Geometry check sheet. Reference: drawing and pictorial views, mm from the part's lowest x, y, z. A direction names the side the tool comes from. Round coordinates to 2 decimals unless told otherwise and drop trailing zeros. Order: outer loops, then holes, each group sorted by start corner. A loop starts at its lowest first (then second) coordinate and runs counter-clockwise, first axis right, second up. Notation, with made-up numbers: (55, 12.25) -> (104, 12.25) arc R33 ccw to (104, 46.25) -> close; hole circle Ø6 at (-40, 82.5). An arc over 180 degrees is marked (long way). Put each result on its own line as item: value.
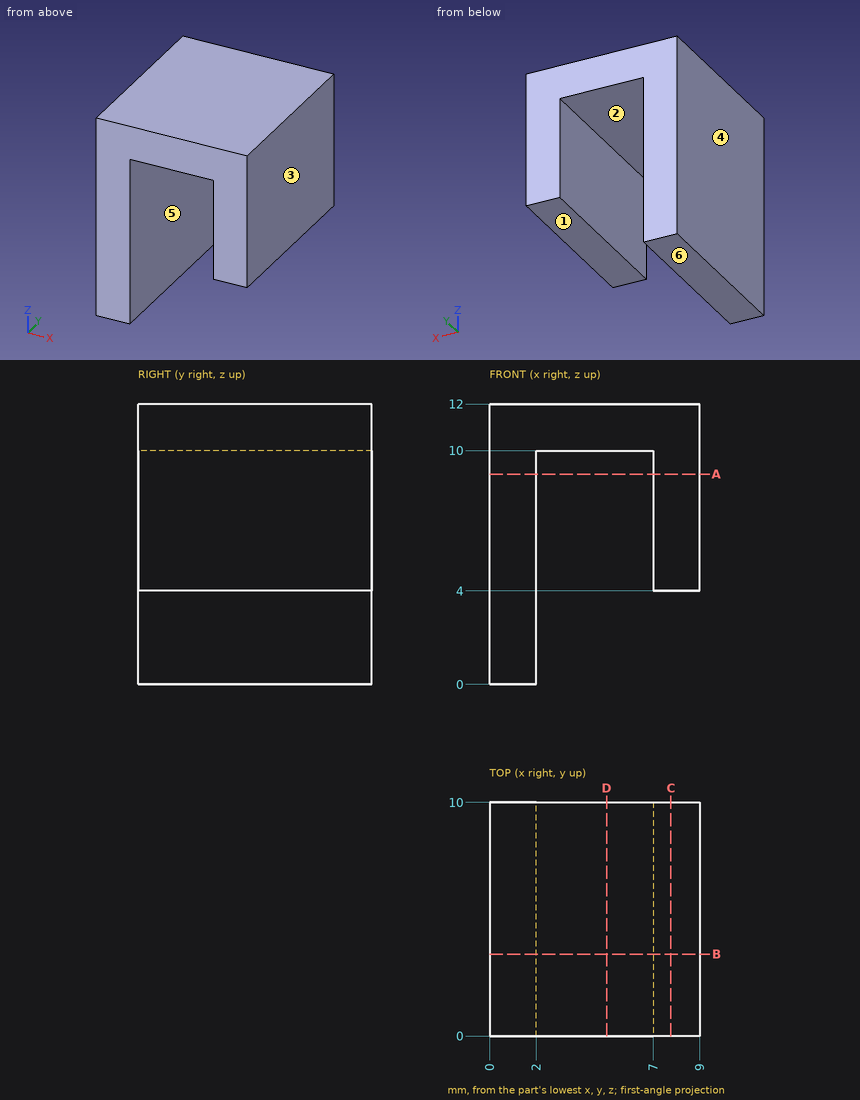
Item 1: Tool access check on the marked faces 5 and 6. Record the directions out of +Z, -Z, +X, -X, +Y, -Y that give a thin tool (end or side, any length) a straight path to the whole face; none if there is none.
Geometry check:
face 5: -Z, +Y, -Y
face 6: -Z, +X, -X, +Y, -Y
Item 2: Release check for a two-part mould opening along X. For the marked faces 1, 2, 3 and 4 record: pulls with the +X half, pulls with the -X half, needs draft (parallel to the pull), parting line crosses it, or undercut.
Geometry check:
face 1: needs draft
face 2: undercut
face 3: pulls with the +X half
face 4: pulls with the -X half
Item 3: Sectioned sample at D-D, the plane x = 5. Record the boundary of the cut face in (y, z).
Geometry check:
outline: (0, 10) -> (10, 10) -> (10, 12) -> (0, 12) -> close
Item 4: Material ranges on line 1 along X through (y, z) = (5.5, 6); line 2 along Z through (x, y) = (2.5, 2.75); line 3 along Z through (x, y) = (8.75, 2.5), recorded low to high.
Geometry check:
line 1: 0 to 2, 7 to 9
line 2: 10 to 12
line 3: 4 to 12
Item 5: Sectioned sample at C-C, the plane x = 7.75. Record the boundary of the cut face in (y, z).
Geometry check:
outline: (0, 4) -> (10, 4) -> (10, 12) -> (0, 12) -> close
Item 6: Sectioned sample at A-A, the plane z = 9. Record the boundary of the cut face in (x, y).
Geometry check:
outline: (0, 0) -> (2, 0) -> (2, 10) -> (0, 10) -> close; (7, 0) -> (9, 0) -> (9, 10) -> (7, 10) -> close
Item 7: Depth check by flat-ended pin: pin 1 Ø0.6 at (x, y) = (7.5, 6) entering from -Z. Enter the tip coordinate at first touch or a pass-through.
Geometry check:
pin 1: z = 4
Item 8: Sectioned sample at B-B, the plane y = 3.5. Record the boundary of the cut face in (x, z).
Geometry check:
outline: (0, 0) -> (2, 0) -> (2, 10) -> (7, 10) -> (7, 4) -> (9, 4) -> (9, 12) -> (0, 12) -> close
